Source: CAD feature listing. Evaluate the final solid. Frame: model axes, mm. Face numbers are marked on the shaded views. A direction names the side the tool comes from. Coordinates: 2 decimals unless noted, no trailing zeros. Order: outer loops, then holes, each group sorted by start corner. A loop starts at its lowest first (then second) coordinate and runs counter-clockwise, first axis right, second up.
```python
from build123d import *

# Parameters (mm, degrees)
BOSS_EXTRUDE1_DEPTH = 5.5
SKETCH2_R           = 1.5
CUT_EXTRUDE2_DEPTH  = 6.5
SKETCH2_4_R         = 3
SKETCH2_4_R_2       = 1.5
CUT_EXTRUDE3_DEPTH  = 1
SKETCH4_R           = 3
CUT_EXTRUDE4_DEPTH  = 1


with BuildPart() as part:
    # Sketch1 → Boss-Extrude1 (new body)
    with BuildSketch(Plane(origin=(0, 0, 0), x_dir=(1, 0, 0), z_dir=(0, 1, 0))):
        with BuildLine():
            Line((0, 5.48), (-0.670562296, 3.888305602))
            ThreePointArc((-0.670562296, 3.888305602), (-0.777902483, 3.74073052), (-0.939622693, 3.656191214))
            ThreePointArc((-0.939622693, 3.656191214), (-1.166539154, 3.590238349), (-1.388884548, 3.510217189))
            ThreePointArc((-1.388884548, 3.510217189), (-1.569409904, 3.483554169), (-1.742992396, 3.53985194))
            Line((-1.742992396, 3.53985194), (-3.221063183, 4.433413129))
            Line((-3.221063183, 4.433413129), (-2.827984983, 2.751558684))
            ThreePointArc((-2.827984983, 2.751558684), (-2.828082561, 2.569074955), (-2.909226002, 2.405624465))
            ThreePointArc((-2.909226002, 2.405624465), (-3.054039154, 2.218889327), (-3.186885098, 2.023459505))
            ThreePointArc((-3.186885098, 2.023459505), (-3.31726105, 1.895778528), (-3.490783235, 1.839295151))
            Line((-3.490783235, 1.839295151), (-5.211789709, 1.693413129))
            Line((-5.211789709, 1.693413129), (-3.905213526, 0.56380987))
            ThreePointArc((-3.905213526, 0.56380987), (-3.798031224, 0.416120077), (-3.76760386, 0.236190934))
            ThreePointArc((-3.76760386, 0.236190934), (-3.775, 0), (-3.76760386, -0.236190934))
            ThreePointArc((-3.76760386, -0.236190934), (-3.798031224, -0.416120077), (-3.905213526, -0.56380987))
            Line((-3.905213526, -0.56380987), (-5.211789709, -1.693413129))
            Line((-5.211789709, -1.693413129), (-3.490783235, -1.839295151))
            ThreePointArc((-3.490783235, -1.839295151), (-3.31726105, -1.895778528), (-3.186885098, -2.023459505))
            ThreePointArc((-3.186885098, -2.023459505), (-3.054039154, -2.218889327), (-2.909226002, -2.405624465))
            ThreePointArc((-2.909226002, -2.405624465), (-2.828082561, -2.569074955), (-2.827984983, -2.751558684))
            Line((-2.827984983, -2.751558684), (-3.221063183, -4.433413129))
            Line((-3.221063183, -4.433413129), (-1.742992396, -3.53985194))
            ThreePointArc((-1.742992396, -3.53985194), (-1.569409904, -3.483554169), (-1.388884548, -3.510217189))
            ThreePointArc((-1.388884548, -3.510217189), (-1.166539154, -3.590238349), (-0.939622693, -3.656191214))
            ThreePointArc((-0.939622693, -3.656191214), (-0.777902483, -3.74073052), (-0.670562296, -3.888305602))
            Line((-0.670562296, -3.888305602), (0, -5.48))
            Line((0, -5.48), (0.670562296, -3.888305602))
            ThreePointArc((0.670562296, -3.888305602), (0.777902483, -3.74073052), (0.939622693, -3.656191214))
            ThreePointArc((0.939622693, -3.656191214), (1.166539154, -3.590238349), (1.388884548, -3.510217189))
            ThreePointArc((1.388884548, -3.510217189), (1.569409904, -3.483554169), (1.742992396, -3.53985194))
            Line((1.742992396, -3.53985194), (3.221063183, -4.433413129))
            Line((3.221063183, -4.433413129), (2.827984983, -2.751558684))
            ThreePointArc((2.827984983, -2.751558684), (2.828082561, -2.569074955), (2.909226002, -2.405624465))
            ThreePointArc((2.909226002, -2.405624465), (3.054039154, -2.218889327), (3.186885098, -2.023459505))
            ThreePointArc((3.186885098, -2.023459505), (3.31726105, -1.895778528), (3.490783235, -1.839295151))
            Line((3.490783235, -1.839295151), (5.211789709, -1.693413129))
            Line((5.211789709, -1.693413129), (3.905213526, -0.56380987))
            ThreePointArc((3.905213526, -0.56380987), (3.798031224, -0.416120077), (3.76760386, -0.236190934))
            ThreePointArc((3.76760386, -0.236190934), (3.775, 0), (3.76760386, 0.236190934))
            ThreePointArc((3.76760386, 0.236190934), (3.798031224, 0.416120077), (3.905213526, 0.56380987))
            Line((3.905213526, 0.56380987), (5.211789709, 1.693413129))
            Line((5.211789709, 1.693413129), (3.490783235, 1.839295151))
            ThreePointArc((3.490783235, 1.839295151), (3.31726105, 1.895778528), (3.186885098, 2.023459505))
            ThreePointArc((3.186885098, 2.023459505), (3.054039154, 2.218889327), (2.909226002, 2.405624465))
            ThreePointArc((2.909226002, 2.405624465), (2.828082561, 2.569074955), (2.827984983, 2.751558684))
            Line((2.827984983, 2.751558684), (3.221063183, 4.433413129))
            Line((3.221063183, 4.433413129), (1.742992396, 3.53985194))
            ThreePointArc((1.742992396, 3.53985194), (1.569409904, 3.483554169), (1.388884548, 3.510217189))
            ThreePointArc((1.388884548, 3.510217189), (1.166539154, 3.590238349), (0.939622693, 3.656191214))
            ThreePointArc((0.939622693, 3.656191214), (0.777902483, 3.74073052), (0.670562296, 3.888305602))
            Line((0.670562296, 3.888305602), (0, 5.48))
        make_face()
    extrude(amount=BOSS_EXTRUDE1_DEPTH)

    # Sketch2 → Cut-Extrude2 (cut, through all)
    with BuildSketch(Plane(origin=(0, 5.5, 0), x_dir=(1, 0, 0), z_dir=(0, 1, 0))):
        Circle(SKETCH2_R)
    extrude(amount=-CUT_EXTRUDE2_DEPTH, mode=Mode.SUBTRACT)

    # Sketch2_4 → Cut-Extrude3 (cut)
    with BuildSketch(Plane(origin=(0, 5.5, 0), x_dir=(1, 0, 0), z_dir=(0, 1, 0))):
        Circle(SKETCH2_4_R)
        Circle(SKETCH2_4_R_2, mode=Mode.SUBTRACT)
    extrude(amount=-CUT_EXTRUDE3_DEPTH, mode=Mode.SUBTRACT)

    # Sketch4 → Cut-Extrude4 (cut)
    with BuildSketch(Plane.XZ):
        Circle(SKETCH4_R)
    extrude(amount=-CUT_EXTRUDE4_DEPTH, mode=Mode.SUBTRACT)


solid = part.part
```
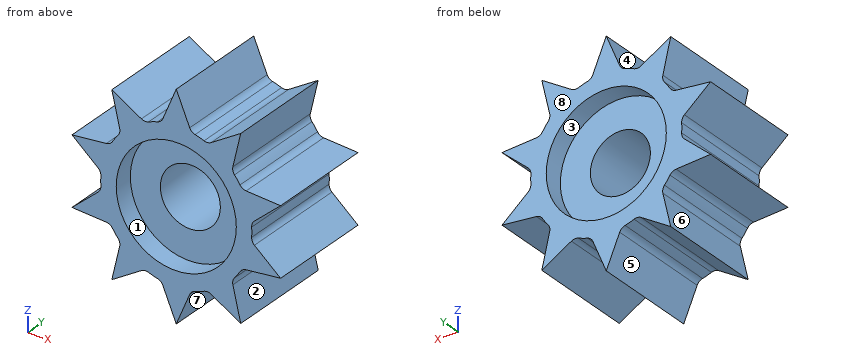
1. Draft query along X for the marked faces 6, 7 and 8. Return one class per face: released by +X, released by -X, zero draft, split by the parting line, or undercut.
Findings:
face 6: released by -X
face 7: undercut
face 8: zero draft
2. Access query for the marked faces 1, 2, 3, 4 and 5. Directions: +Z, -Z, +X, -X, +Y, -Y. A direction counts if a zero-diameter tool reaches every point of the face in a straight line with its end or side. Return the directions, or none.
Findings:
face 1: -Y
face 2: +X, +Y, -Y
face 3: +Y
face 4: +Z, +Y, -Y
face 5: -Z, +Y, -Y
3. Section query A-A on z = 0. Return loops of the section in (x, y) (3 decimals), plus the area to 3 significant figures.
Findings:
outline: (-3.775, 0) - (-3, 0) - (-3, 1) - (-1.5, 1) - (-1.5, 4.5) - (-3, 4.5) - (-3, 5.5) - (-3.775, 5.5) - close; (1.5, 1) - (3, 1) - (3, 0) - (3.775, 0) - (3.775, 5.5) - (3, 5.5) - (3, 4.5) - (1.5, 4.5) - close
area: 19.0 mm2
4. Ray query, line 1 (X direction, y = 2.85, z = 0) (3 decimals); line 2 (X direction, y = 5, z = 0) (3 decimals); line 3 (Z direction, x = 3.5, y = 2.4). Return the intervals inside material, ascending.
Findings:
line 1: x = -3.775 to -1.5, 1.5 to 3.775
line 2: x = -3.775 to -3, 3 to 3.775
line 3: z = -1.84 to 1.84
5. Section query B-B on x = 2.25. Return loops of the section in (y, z), plus the area to 3 significant figures.
Findings:
outline: (0, -3.85) - (5.5, -3.85) - (5.5, -1.98) - (4.5, -1.98) - (4.5, 1.98) - (5.5, 1.98) - (5.5, 3.85) - (0, 3.85) - (0, 1.98) - (1, 1.98) - (1, -1.98) - (0, -1.98) - close
area: 34.4 mm2
6. Pin query (flat end, axial travel): P1, Ø2, axis at x = 2.5, y = 1, coming from the +Z side; P2, Ø1.5, axis at y = 1.5, z = -3.5, coming from the +X side; P3, Ø5.5, axis at x = 0, z = 0, coming from the -Y side. Return the tip coordinate at first contact, or that it passes through.
Findings:
P1: stops at z = 4.43
P2: stops at x = 3.18
P3: stops at y = 1
